Read the model definition and answer for the solid it produces. Units are mm, in the model's axes. A direction names the side the tool comes from. Coordinates: 2 decimals unless noted, no trailing zeros. Order: outer loops, then holes, each group sorted by start corner. A loop starts at its lowest first (then second) coordinate and runs counter-clockwise, first axis right, second up.
```python
from build123d import *

# Parameters (mm, degrees)
F0_W     = 15
F0_H     = 2
F0_R     = 0.5
F1_DEPTH = 3
F2_R     = 1.5
F3_DEPTH = 5


with BuildPart() as f1:
    # F0 (on Front) → F1 (new body)
    with BuildSketch(Plane.XZ):
        with Locations((-1.4090953767, 14.3183305617)):
            Rectangle(F0_W, F0_H)
        with Locations((5.0909046233, 14.3183305617)):
            Circle(F0_R, mode=Mode.SUBTRACT)
        Polygon((-8.9090953767, 13.3183305617), (-8.9090953767, 15.3183305617), (-16.4090953767, 12.3621613234), (-16.4090953767, 10.3621613234), align=None)
    extrude(amount=F1_DEPTH)

    # F2 (on face) → F3 (join)
    with BuildSketch(Plane(origin=(-5.7415974535, 0, 14.5668185514), x_dir=(0.9303396878, 0, 0.3666988755), z_dir=(0.3666988755, 0, -0.9303396878))):
        with Locations((-9.9662397649, 1.5)):
            Circle(F2_R)
    extrude(amount=F3_DEPTH)


solid = f1.part
```
1) A cutting plane is placed at A-A, the plane y = -0.45. Determine the outline of the cut face in (x, z), and give its area (3 significant figures).
A:
outline: (-16.41, 10.36) - (-16.01, 10.52) - (-14.18, 5.87) - (-12.18, 6.65) - (-14.02, 11.31) - (-8.91, 13.32) - (6.09, 13.32) - (6.09, 15.32) - (-8.91, 15.32) - (-16.41, 12.36) - close; hole circle Ø1 at (5.09, 14.32)
area: 54.9 mm2
2) A cutting plane is placed at C-C, the plane x = -2.5. Determine the outline of the cut face in (y, z).
A:
outline: (-3, 13.32) - (0, 13.32) - (0, 15.32) - (-3, 15.32) - close
3) Which of the six approach directions +Z, -Z, +X, -X, +Y, -Y give full straight-line access (tool end or side, diameter ignored) to faces 5 (the flat face through (-2, -1, 13.318)), 6 (the cylindrical face through (-12.779, -1.951, 9.144)), 7 (the flat face through (-16.128, -2.635, 10.473))?
A:
face 5: -Z, +X, +Y, -Y
face 6: none
face 7: -Z, -Y
4) A cutting plane is placed at B-B, the plane y = -2.05. Determine the outline of the cut face in (x, z), and give its area (3 significant figures).
A:
outline: (-16.41, 10.36) - (-16.31, 10.4) - (-14.48, 5.75) - (-11.88, 6.77) - (-13.72, 11.42) - (-8.91, 13.32) - (6.09, 13.32) - (6.09, 15.32) - (-8.91, 15.32) - (-16.41, 12.36) - close; hole circle Ø1 at (5.09, 14.32)
area: 58.2 mm2
5) Straight lines are drawn through the part: line 1 (Z direction, x = -2.25, y = -1.1); line 2 (X direction, y = -1.2, z = 9); line 3 (X direction, y = -0.9, z = 10.75). For each, find the intervals that lie inside material, in ascending order.
A:
line 1: z = 13.32 to 15.32
line 2: x = -15.84 to -12.68
line 3: x = -16.41 to -13.47
6) A flat-ended cylindrical pin translates along its axis: pin 1 Ø1 at (y, z) = (-2.5, 9.5) entering from +X. Find the tip coordinate at first contact, or state that the pin passes through.
A:
pin 1: stops at x = -12.86
7) Determine the mould class of faces 1 (the flat face through (-12.61, -1.48, 13.86)), 2 (the cylindrical face through (4.98, -1.48, 13.83)), 3 (the flat face through (-16.128, -0.358, 10.473)), 4 (the flat face through (-2, -1, 15.318)) for opening direction X: pulls with the +X half, pulls with the -X half, needs draft (parallel to the pull), parting line crosses it, or undercut.
A:
face 1: pulls with the -X half
face 2: undercut
face 3: undercut
face 4: needs draft
8) A cutting plane is placed at D-D, the plane z = 12.75. Determine the outline of the cut face in (x, y).
A:
outline: (-15.43, -3) - (-10.35, -3) - (-10.35, 0) - (-15.43, 0) - close
